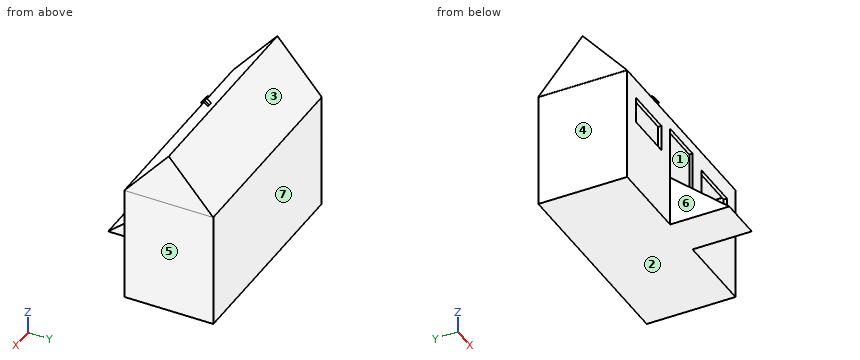
from build123d import *

# Parameters (mm, degrees)
F0_W      = 44.3399958313
F0_H      = 14.4718540832
F1_DEPTH  = 38.1
F2_W      = 34.0127944946
F2_H      = 1.2406939641
F2_W_2    = 18.4130221605
F3_DEPTH  = 25.4
F4_W      = 20.9599845111
F4_H      = 11.3026611507
F5_DEPTH  = 25.4
F6_W      = 18.4130221605
F6_H      = 1.415140456
F7_DEPTH  = 2.54
F8_W      = 18.4130221605
F8_H      = 21.8460503966
F9_DEPTH  = 25.4
F11_DEPTH = 25.4
F12_W     = 88.6799916625
F12_H     = 38.1
F13_DEPTH = 2.54
F15_DEPTH = 44.45
F16_W     = 31.7063815892
F16_H     = 38.1
F17_DEPTH = 25.4
F18_W     = 1.5490213409
F18_H     = 0.9214421734
F19_DEPTH = 2.54
F20_W     = 0.7745106705
F20_H     = 0.4545422271
F20_H_2   = 0.4668999463
F21_DEPTH = 0.254


with BuildPart() as f1:
    # F0 (on Front) → F1 (new body)
    with BuildSketch(Plane.XZ):
        with Locations((22.1699979156, -7.2359270416)):
            Rectangle(F0_W, F0_H)
        with Locations((-22.1699979156, -7.2359270416)):
            Rectangle(F0_W, F0_H)
        Polygon((44.3399958313, -14.4718540832), (0, -14.4718540832), (-44.3399958313, -14.4718540832), (-76.0463774204, -14.4718540832), (-76.0463774204, -21.8460503966), (0, -21.8460503966), (76.0463774204, -21.8460503966), (76.0463774204, -14.4718540832), align=None)
    extrude(amount=F1_DEPTH)

    # F2 (on face) → F3 (join)
    with BuildSketch(Plane.XY):
        with Locations((-26.2129083276, -0.620346982)):
            Rectangle(F2_W, F2_H)
        with Locations((0, -0.620346982)):
            Rectangle(F2_W_2, F2_H)
        with Locations((26.2129083276, -0.620346982)):
            Rectangle(F2_W, F2_H)
        Polygon((-43.2193055749, -1.2406939641), (-43.2193055749, 0), (-44.3399958313, 0), (-44.3399958313, -36.684859544), (-43.2193055749, -36.684859544), align=None)
        Polygon((-44.3399958313, -38.1), (-9.2065110803, -38.1), (-9.2065110803, -36.684859544), (-43.2193055749, -36.684859544), (-44.3399958313, -36.684859544), align=None)
        Polygon((44.3399958313, -38.1), (44.3399958313, -36.684859544), (43.2193055749, -36.684859544), (9.2065110803, -36.684859544), (9.2065110803, -38.1), align=None)
        Polygon((44.3399958313, -36.684859544), (44.3399958313, 0), (43.2193055749, 0), (43.2193055749, -1.2406939641), (43.2193055749, -36.684859544), align=None)
    extrude(amount=F3_DEPTH)

    # F4 (on face) → F5 (cut)
    with BuildSketch(Plane.XZ.offset(38.1)):
        with Locations((-26.8112961203, 14.027569443)):
            Rectangle(F4_W, F4_H)
        with Locations((26.8112961203, 14.027569443)):
            Rectangle(F4_W, F4_H)
    extrude(amount=-F5_DEPTH, mode=Mode.SUBTRACT)

    # F6 (on face) → F7 (join)
    with BuildSketch(Plane.XY.offset(25.4)):
        with Locations((0, -37.392429772)):
            Rectangle(F6_W, F6_H)
    extrude(amount=-F7_DEPTH)

    # F8 (on face) → F9 (join)
    with BuildSketch(Plane.XZ.offset(38.1)):
        with Locations((0, -10.9230251983)):
            Rectangle(F8_W, F8_H)
    extrude(amount=F9_DEPTH)

    # F10 (on face) → F11 (cut)
    with BuildSketch(Plane(origin=(-9.2065110803, 0, 0), x_dir=(0, -1, 0), z_dir=(-1, 0, 0))):
        Polygon((63.5, 0), (38.1, 0), (63.5, -21.8460503966), align=None)
    extrude(amount=-F11_DEPTH, mode=Mode.SUBTRACT)

    # F12 (on face) → F13 (join)
    with BuildSketch(Plane.XY.offset(25.4)):
        with Locations((0, -19.05)):
            Rectangle(F12_W, F12_H)
    extrude(amount=F13_DEPTH)

    # F14 (on Right) → F15 (join, symmetric)
    with BuildSketch(Plane.YZ):
        Polygon((-38.1, 27.94), (-19.05, 27.94), (-19.05, 50.1542687416), align=None)
        Polygon((-19.05, 27.94), (0, 27.94), (-19.05, 50.1542687416), align=None)
    extrude(amount=F15_DEPTH, both=True)

    # F16 (on face) → F17 (cut)
    with BuildSketch(Plane.XY.offset(-14.4718540832)):
        with Locations((60.1931866258, -19.05)):
            Rectangle(F16_W, F16_H)
        with Locations((-60.1931866258, -19.05)):
            Rectangle(F16_W, F16_H)
    extrude(amount=-F17_DEPTH, mode=Mode.SUBTRACT)

    # F18 (on face) → F19 (join)
    with BuildSketch(Plane(origin=(0, -35.7612087902, 30.6672722554), x_dir=(1, 0, 0), z_dir=(0, -0.7591012698, 0.650972551))):
        with Locations((-4.9122394994, 12.6880933531)):
            Rectangle(F18_W, F18_H)
    extrude(amount=F19_DEPTH)

    # F20 (on face) → F21 (join)
    with BuildSketch(Plane(origin=(0, -37.6893260156, 32.3207425348), x_dir=(1, 0, 0), z_dir=(0, -0.7591012698, 0.650972551))):
        Polygon((-5.6867501698, 13.1488144398), (-4.9122394994, 13.1488144398), (-4.9122394994, 13.6726424098), (-6.5931216814, 13.6726424098), (-6.5931216814, 12.6819144934), (-5.6867501698, 12.6819144934), align=None)
        Polygon((-4.9122394994, 13.1488144398), (-4.1377288289, 13.1488144398), (-4.1377288289, 12.6819144934), (-3.2313573174, 12.6819144934), (-3.2313573174, 13.6726424098), (-4.9122394994, 13.6726424098), align=None)
        Polygon((-3.2313573174, 12.6819144934), (-4.1377288289, 12.6819144934), (-4.1377288289, 12.2273722664), (-4.9122394994, 12.2273722664), (-4.9122394994, 11.6911865771), (-3.2313573174, 11.6911865771), align=None)
        with Locations((-5.2994948346, 12.4546433799)):
            Rectangle(F20_W, F20_H)
        with Locations((-5.2994948346, 12.9153644666)):
            Rectangle(F20_W, F20_H_2)
        with Locations((-4.5249841642, 12.9153644666)):
            Rectangle(F20_W, F20_H_2)
        with Locations((-4.5249841642, 12.4546433799)):
            Rectangle(F20_W, F20_H)
        Polygon((-5.6867501698, 12.2273722664), (-5.6867501698, 12.6819144934), (-6.5931216814, 12.6819144934), (-6.5931216814, 11.6911865771), (-4.9122394994, 11.6911865771), (-4.9122394994, 12.2273722664), align=None)
    extrude(amount=F21_DEPTH)


solid = f1.part
Design review of the part built by this model. Coordinates are the model's own, in mm. Face numbers are marked on the shaded views. A direction names the side the tool comes from. Give positions to 0.01 mm unless a question says otherwise; leave off trailing zeros. Write each loop counter-clockwise with the first axis right and the second up, starting at its lowest first coordinate (ties: lowest second). Pieces come first, ordered by that corner, then holes. Notation, with made-up numbers: M 76.5,11.25 L 83.5,11.25 A22 ccw 83.5,43.25 Z; hole C 62.25,-18 d5. An arc over 180 degrees is marked long. Answer as a JSON object with one key per item and string values. Group by question number.
1) Clearance check with flat-ended pins moving along their axes: pin 1 Ø0.7 at (x, y) = (30, -37.5) entering from +Z; pin 2 Ø11.5 at (y, z) = (-14, -7.5) entering from +X; pin 3 Ø2.5 at (y, z) = (-28.5, 41.5) entering from +X. State where each tip first meets the part, or that it passes through.
2) For line 1 along Y through (x, z) = (40, 1); line 2 along X through (y, z) = (-30.5, 16.5); line 3 along Z through (x, y) = (14.5, -19.5), list the stretches that pass through material, from the lowest coordinate up.
3) We need section A-A (z = 17). Give the boundary of the cut face in (x, y), and give its area (3 significant figures).
4) We need section B-B (x = 24.5). Give the boundary of the cut face in (y, z).
5) Mouldability with a two-part tool opening along Z and no side actions: class the marked faces 1, 2, 3 and 4 as released by +Z, released by -Z, zero draft, split by the parting line, or undercut.
6) We need section C-C (y = -5.5). Give the boundary of the cut face in (x, z).
7) We need section D-D (z = -16). Give the boundary of the cut face in (x, y), and give its area (3 significant figures).
8) Tool access review of the marked faces 5, 6 and 7: name each direction out of +Z, -Z, +X, -X, +Y, -Y from which nothing blocks a thin tool from reaching the whole face with its end or side.
Answer key:
{
 "1": {"pin 1": "stops at z = 29.05", "pin 2": "stops at x = 44.34", "pin 3": "stops at x = -3.23"},
 "2": {"line 1": "y = -38.1 to -36.68, -1.24 to 0", "line 2": "x = -44.34 to -43.22, 43.22 to 44.34", "line 3": "z = -21.85 to 0, 25.4 to 49.63"},
 "3": {"outline": "M -44.34,-38.1 L -37.29,-38.1 L -37.29,-36.68 L -43.22,-36.68 L -43.22,-1.24 L 43.22,-1.24 L 43.22,-36.68 L 37.29,-36.68 L 37.29,-38.1 L 44.34,-38.1 L 44.34,0 L -44.34,0 Z; M -16.33,-38.1 L -9.21,-38.1 L -9.21,-36.68 L -16.33,-36.68 Z; M 9.21,-38.1 L 16.33,-38.1 L 16.33,-36.68 L 9.21,-36.68 Z", "area": "230 mm²"},
 "4": {"outline": "M -38.1,-21.85 L 0,-21.85 L 0,27.94 L -19.05,50.15 L -38.1,27.94 L -38.1,19.68 L -36.68,19.68 L -36.68,25.4 L -1.24,25.4 L -1.24,0 L -36.68,0 L -36.68,8.38 L -38.1,8.38 Z"},
 "5": {"face 1": "undercut", "face 2": "released by -Z", "face 3": "released by +Z", "face 4": "zero draft"},
 "6": {"outline": "M -44.45,27.94 L -44.34,27.94 L -44.34,-21.85 L 44.34,-21.85 L 44.34,27.94 L 44.45,27.94 L 44.45,34.35 L -44.45,34.35 Z; hole M -43.22,0 L 43.22,0 L 43.22,25.4 L -43.22,25.4 Z"},
 "7": {"outline": "M -44.34,-38.1 L -9.21,-38.1 L -9.21,-56.7 L 9.21,-56.7 L 9.21,-38.1 L 44.34,-38.1 L 44.34,0 L -44.34,0 Z", "area": "3,720 mm²"},
 "8": {"face 5": "-Z, +X, +Y, -Y", "face 6": "+Z, -Z, -X, -Y", "face 7": "+Z, -Z, +X, -X, +Y"}
}
